Autodesk Inventor part; units mm, degrees
ref_plane "YZ Plane" through (0, 0, 0) normal (1, 0, 0) x (0, 1, 0)
ref_plane "XZ Plane" through (0, 0, 0) normal (0, 1, 0) x (-1, 0, 0)
ref_plane "XY Plane" through (0, 0, 0) normal (0, 0, 1) x (1, 0, 0)
sketch "Szkic1" plane through (0, 0, 0) normal (0, 1, 0) x (-1, 0, 0)
  line L0 (-27.5, -37.75) -> (27.5, -37.75)
  line L1 (27.5, -37.75) -> (27.5, 37.75)
  line L2 (27.5, 37.75) -> (-27.5, 37.75)
  line L3 (-27.5, 37.75) -> (-27.5, -37.75)
  line L4 (-27.5, -37.75) -> (27.5, 37.75) construction
  line L5 (27.5, -37.75) -> (-27.5, 37.75) construction
  point P0 (0, 0)
  dimension "d0" = 55
  dimension "d1" = 75.5
extrude "Wyciągnięcie proste1" add sketch "Szkic1" along normal blind 2
sketch "Szkic2" plane through (0, 0, 0) normal (0, -1, 0) x (1, 0, 0)
  line L0 (15.75, -7.5) -> (15.75, -11.75)
  line L1 (15.75, -11.75) -> (13, -11.75)
  arc A0 (13, -11.75) -> (13, -17.25) centre (13, -14.5) ccw
  line L2 (13, -17.25) -> (15.75, -17.25)
  line L3 (15.75, -17.25) -> (15.75, -21.5)
  line L4 (15.75, -21.5) -> (-20.25, -21.5)
  line L5 (-20.25, -21.5) -> (-20.25, -17.25)
  line L6 (-20.25, -17.25) -> (-17.5, -17.25)
  arc A1 (-17.5, -17.25) -> (-17.5, -11.75) centre (-17.5, -14.5) ccw
  line L7 (-17.5, -11.75) -> (-20.25, -11.75)
  line L8 (-20.25, -11.75) -> (-20.25, -7.5)
  line L9 (-20.25, -7.5) -> (15.75, -7.5)
  circle A2 centre (-17.5, -14.5) radius 1.75
  circle A3 centre (19.25, -34.5) radius 1.75
  circle A4 centre (-23.75, 34.5) radius 1.75
  circle A5 centre (-23.75, -34.5) radius 1.75
  circle A6 centre (19.25, 34.5) radius 1.75
  circle A7 centre (13, -14.5) radius 1.75
  line L10 (23, -37.75) -> (-27.5, -37.75)
  line L11 (23, 37.75) -> (23, -37.75)
  line L12 (-27.5, 37.75) -> (23, 37.75)
  line L13 (-27.5, -37.75) -> (-27.5, 37.75)
  line L14 (-20.25, -21.5) -> (15.75, -21.5)
  point P0 (0, 0)
hole "Otwór1" at (19.25, 0, 34.5) at (19.25, 0, -34.5) at (13, 0, -14.5) at (-17.5, 0, -14.5) at (-23.75, 0, -34.5) at (-23.75, 0, 34.5) direction (0, 1, 0) diameter 3.5 end through all
properties part number "blacha pionowa ste driver"
Read the model definition and answer for the solid it produces. Units are mm, in the model's axes. Coordinates: 2 decimals unless noted, no trailing zeros. Write each loop counter-clockwise with the first axis right and the second up, starting at its lowest first coordinate (ties: lowest second). Pieces come first, ordered by that corner, then holes. Notation, with made-up numbers: M 15,-18.75 L 36,-18.75 A30 cw 36,9.25 Z; hole C 25.25,-23.5 d9. An arc over 180 degrees is marked long. Use a Markdown table: item, result.
Q1. The part is cut by section C-C, the plane x = 13. Write down the section's boundary in (y, z), then the cut area to 3 significant figures.
Answer block:
| item | result |
|---|---|
| outline | M 0,-37.75 L 2,-37.75 L 2,-16.25 L 0,-16.25 Z; M 0,-12.75 L 2,-12.75 L 2,37.75 L 0,37.75 Z |
| area | 144 mm2 |
Q2. Straight lines are drawn through the part: L1, parallel to X at y = 1.6, z = -34.5; L2, parallel to X at y = 0.9, z = -14.5; L3, parallel to Z at x = -23.75, y = 1.15. For each, find the intervals that lie inside material, in ascending order. Write a range as [from, to].
Answer block:
| item | result |
|---|---|
| L1 | x = [-27.5, -25.5], [-22, 17.5], [21, 27.5] |
| L2 | x = [-27.5, -19.25], [-15.75, 11.25], [14.75, 27.5] |
| L3 | z = [-37.75, -36.25], [-32.75, 32.75], [36.25, 37.75] |
Q3. This flat-tipped pin is pushed along its axis until it touches: pin 1 Ø2 at (x, z) = (13, -14.5) entering from -Y. Where does it stop, or does it pass through?
Answer block:
| item | result |
|---|---|
| pin 1 | passes through |
Q4. The part is cut by section A-A, the plane z = -14.5. Write down the section's boundary in (x, y).
Answer block:
| item | result |
|---|---|
| outline | M -27.5,0 L -19.25,0 L -19.25,2 L -27.5,2 Z; M -15.75,0 L 11.25,0 L 11.25,2 L -15.75,2 Z; M 14.75,0 L 27.5,0 L 27.5,2 L 14.75,2 Z |
Q5. The part is cut by section B-B, the plane x = -23.75. Write down the section's boundary in (y, z).
Answer block:
| item | result |
|---|---|
| outline | M 0,-37.75 L 2,-37.75 L 2,-36.25 L 0,-36.25 Z; M 0,-32.75 L 2,-32.75 L 2,32.75 L 0,32.75 Z; M 0,36.25 L 2,36.25 L 2,37.75 L 0,37.75 Z |
Q6. Determine the mould class of faces 1 (the face through (-24.93, 1.01, 35.79)), 2 (the face through (0, 2, 1)), 3 (the face through (11.265, 1.014, -14.272)), 4 (the face through (0, 1, 37.75)) for opening direction Z: released by +Z, released by -Z, zero draft, split by the parting line, or undercut.
Answer block:
| item | result |
|---|---|
| face 1 | undercut |
| face 2 | zero draft |
| face 3 | undercut |
| face 4 | released by +Z |
